For this review, take the finished solid that the model builds, in its own axes (mm). Give positions to 0.01 mm unless a question says otherwise; leave off trailing zeros. Write each loop counter-clockwise with the first axis right and the second up, starting at its lowest first coordinate (ties: lowest second). Pieces come first, ordered by that corner, then holes. Notation, with made-up numbers: M -19,50.25 L 37,50.25 A10 cw 37,57.25 Z; hole C 40.25,13.5 d10. An arc over 180 degrees is marked long. One line per item, written item: value. Start each with the question number.
Item 1: Clearance check with a flat-ended pin moving along its axis: pin 1 Ø5.5 at (x, z) = (193.675, -136.525) entering from +Y. State where the tip first meets the part, or that it passes through.
Item 2: To check wall thickness, follow probe 1 along X at (y, z) = (3.75, 193) (3 decimals); probe 2 along Z at (x, y) = (126.5, 4.5) (3 decimals). State the ranges of each line that lie inside material, in increasing order.
Item 3: Consider section B-B, the plane y = 2.75. Give the number of separate pieces and of enclosed holes in the cut face, and give its area (3 significant figures).
Item 4: Consider section A-A, the plane x = 97.5. Write out the cut boundary in (y, z) (3 decimals).
```python
from build123d import *

# Parameters (mm, degrees)
SKETCH1_W           = 425.45
SKETCH1_H           = 425.45
BOSS_EXTRUDE1_DEPTH = 6.35
SKETCH4_R           = 4.445
CUT_EXTRUDE2_DEPTH  = 301.90558943
SKETCH5_W           = 102.616
SKETCH5_H           = 102.616
CUT_EXTRUDE3_DEPTH  = 301.90558943
FILLET1_R           = 12.7


with BuildPart() as part:
    # Sketch1 → Boss-Extrude1 (new body)
    with BuildSketch(Plane(origin=(0, 0, 0), x_dir=(1, 0, 0), z_dir=(0, 1, 0))):
        Rectangle(SKETCH1_W, SKETCH1_H)
    extrude(amount=BOSS_EXTRUDE1_DEPTH)

    # Sketch4 → Cut-Extrude2 (cut, through all)
    with BuildSketch(Plane(origin=(0, 6.35, 0), x_dir=(1, 0, 0), z_dir=(0, 1, 0))):
        with Locations(Location((-193.675, 136.525, 0), (0, 0, 270))):
            Circle(SKETCH4_R)
        with Locations(Location((-193.675, -136.525, 0), (0, 0, 270))):
            Circle(SKETCH4_R)
        with Locations(Location((-136.525, -193.675, 0), (0, 0, 270))):
            Circle(SKETCH4_R)
        with Locations(Location((136.525, -193.675, 0), (0, 0, 270))):
            Circle(SKETCH4_R)
        with Locations(Location((193.675, -136.525, 0), (0, 0, 90))):
            Circle(SKETCH4_R)
        with Locations(Location((193.675, 136.525, 0), (0, 0, 90))):
            Circle(SKETCH4_R)
        with Locations(Location((136.525, 193.675, 0), (0, 0, 90))):
            Circle(SKETCH4_R)
        with Locations(Location((-136.525, 193.675, 0), (0, 0, 90))):
            Circle(SKETCH4_R)
    extrude(amount=-CUT_EXTRUDE2_DEPTH, mode=Mode.SUBTRACT)

    # Sketch5 → Cut-Extrude3 (cut, through all)
    with BuildSketch(Plane(origin=(0, 6.35, 0), x_dir=(1, 0, 0), z_dir=(0, 1, 0))):
        with Locations((111.125, -111.125)):
            Rectangle(SKETCH5_W, SKETCH5_H)
    extrude(amount=-CUT_EXTRUDE3_DEPTH, mode=Mode.SUBTRACT)

    # Fillet1
    fillet1_edges = [part.edges().sort_by_distance(p)[0] for p in [
        (212.725, 3.175, 212.725),
        (-212.725, 3.175, 212.725),
        (-212.725, 3.175, -212.725),
        (212.725, 3.175, -212.725),
    ]]
    fillet(fillet1_edges, radius=FILLET1_R)


solid = part.part
```
Model answer:
1. pin 1: passes through
2. probe 1: x = -212.725 to -140.918, -132.132 to 132.132, 140.918 to 212.725
2. probe 2: z = -212.725 to 59.817, 162.433 to 212.725
3. separate pieces: 1
3. enclosed holes: 9
3. area: 170,000 mm2
4. outline: M 0,-212.725 L 6.35,-212.725 L 6.35,59.817 L 0,59.817 Z; M 0,162.433 L 6.35,162.433 L 6.35,212.725 L 0,212.725 Z
